Check sheet for the modelled part. Datum: model origin and axes. Units: mm. Face numbers are marked on the shaded views. A direction names the side the tool comes from. Round coordinates to 2 decimals unless told otherwise and drop trailing zeros. Write each loop counter-clockwise with the first axis right and the second up, starting at its lowest first coordinate (ties: lowest second). Pieces come first, ordered by that corner, then holes.
Item 1: Cross-section at D-D on z = -4.5. Enter the section's corners in (x, y).
Item 2: Material ranges on line 1 (Y direction, x = 0.5, z = 0); line 2 (X direction, y = -3.5, z = -0.5); line 3 (Y direction, x = 0, z = -1.25), recorded low to high.
Item 3: Tool access check on the marked faces 4, 5 and 6. Record the directions out of +Z, -Z, +X, -X, +Y, -Y that give a thin tool (end or side, any length) a straight path to the whole face; none if there is none.
Item 4: Cross-section at C-C on x = 6.25. Enter the section's corners in (y, z), plus the area to 3 significant figures.
Item 5: Cross-section at A-A on y = -18.4. Enter the section's corners in (x, z), plus the area to 3 significant figures.
Item 6: Release check for a two-part mould opening along Z. For the marked faces 1, 2 and 3 record: +Z half, -Z half, draft (parallel to the pull), parting line (faces both ways), or undercut.
Item 7: Go/stop test with flat-tipped pins: pin 1 Ø1.6 at (x, z) = (-0.5, 0.5) entering from +Y; pin 2 Ø1.6 at (x, y) = (-0.5, -14) entering from +Z; pin 3 Ø1.6 at (x, y) = (0, -21.5) entering from -Z. Record where each tip stops, or that it passes through.
Item 8: Cross-section at B-B on z = 0. Enter the section's corners in (x, y), plus the area to 3 significant figures.
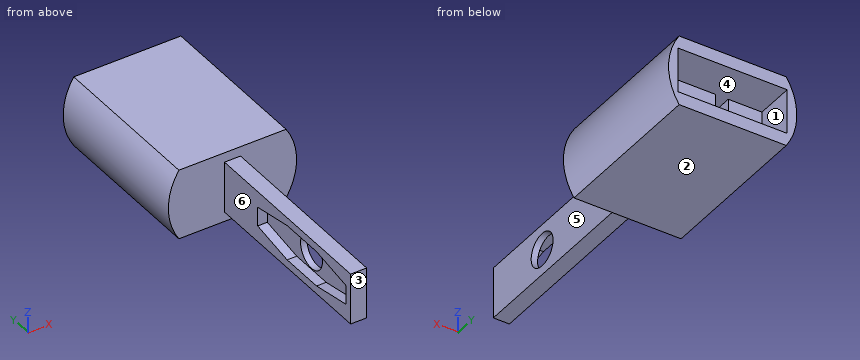
from build123d import *

# Parameters (mm, degrees)
SKETCH3_R           = 10
BOSS_EXTRUDE1_DEPTH = 25
SKETCH4_W           = 2.5
SKETCH4_H           = 8
BOSS_EXTRUDE2_DEPTH = 30
CUT_EXTRUDE1_REACH  = 35.564
SKETCH5_R           = 2.6
SKETCH7_W           = 17
SKETCH7_H           = 7
CUT_EXTRUDE3_DEPTH  = 6
SKETCH8_W           = 2
SKETCH8_H           = 7
CUT_EXTRUDE4_DEPTH  = 4
SKETCH11_W          = 5.5
SKETCH11_H          = 21
CUT_EXTRUDE7_DEPTH  = 1.5
CUT_EXTRUDE5_DEPTH  = 43
BOSS_EXTRUDE3_DEPTH = 1.5


with BuildPart() as part:
    # Sketch3 → Boss-Extrude1 (new body)
    with BuildSketch(Plane(origin=(0, 0, 0), x_dir=(1, 0, 0), z_dir=(0, 1, 0))):
        with Locations(Location((0, 0, 0), (0, 0, 270))):
            Circle(SKETCH3_R)
    extrude(amount=BOSS_EXTRUDE1_DEPTH)

    # Sketch4 → Boss-Extrude2 (add)
    with BuildSketch(Plane(origin=(0, 0, 0), x_dir=(-1, 0, 0), z_dir=(0, -1, 0))):
        Rectangle(SKETCH4_W, SKETCH4_H)
    extrude(amount=BOSS_EXTRUDE2_DEPTH)

    # Sketch5 → Cut-Extrude1 (cut, up to next)
    with BuildSketch(Plane(origin=(1.25, 0, 0), x_dir=(0, 0, -1), z_dir=(1, 0, 0)), mode=Mode.PRIVATE) as cut_extrude1_sk1:
        with Locations((0, -18.4)):
            Circle(SKETCH5_R)
    cut_extrude1_tool1 = extrude(cut_extrude1_sk1.sketch, amount=-CUT_EXTRUDE1_REACH, mode=Mode.PRIVATE) & part.part
    add(cut_extrude1_tool1.solids().sort_by_distance((1.25, -18.4, 0))[0], mode=Mode.SUBTRACT)

    # Sketch7 → Cut-Extrude3 (cut)
    with BuildSketch(Plane(origin=(0, 25, 0), x_dir=(1, 0, 0), z_dir=(0, 1, 0))):
        Rectangle(SKETCH7_W, SKETCH7_H)
    extrude(amount=-CUT_EXTRUDE3_DEPTH, mode=Mode.SUBTRACT)

    # Sketch8 → Cut-Extrude4 (cut)
    with BuildSketch(Plane(origin=(0, 19, 0), x_dir=(1, 0, 0), z_dir=(0, 1, 0))):
        with Locations((-2.25, 0)):
            Rectangle(SKETCH8_W, SKETCH8_H)
    extrude(amount=-CUT_EXTRUDE4_DEPTH, mode=Mode.SUBTRACT)

    # Sketch11 → Cut-Extrude7 (cut)
    with BuildSketch(Plane.ZY.offset(1.25)):
        with Locations((0, -18.4)):
            Rectangle(SKETCH11_W, SKETCH11_H)
    extrude(amount=-CUT_EXTRUDE7_DEPTH, mode=Mode.SUBTRACT)

    # Sketch9 → Cut-Extrude5 (cut)
    with BuildSketch(Plane.XZ):
        with BuildLine():
            Line((8.351646544, -5.5), (-8.351646544, -5.5))
            ThreePointArc((-8.351646544, -5.5), (0, -10), (8.351646544, -5.5))
        make_face()
        with BuildLine():
            Line((8.351646544, 5.5), (-8.351646544, 5.5))
            ThreePointArc((-8.351646544, 5.5), (0, 10), (8.351646544, 5.5))
        make_face()
    extrude(amount=-CUT_EXTRUDE5_DEPTH, mode=Mode.SUBTRACT)

    # Sketch10 → Boss-Extrude3 (add)
    with BuildSketch(Plane.ZY.offset(1.25)):
        Polygon((-2.749970665, -28.900023923), (-2.749970665, -21.900023923), (-1.499970665, -28.900023923), align=None)
        Polygon((1.499970665, -28.900023923), (2.749970665, -28.900023923), (2.749970665, -21.900023923), align=None)
        Polygon((2.749970665, -7.899976077), (2.749970665, -14.899976077), (1.499970665, -7.899976077), align=None)
        Polygon((-1.499970665, -7.899976077), (-2.749970665, -7.899976077), (-2.749970665, -14.899976077), align=None)
    extrude(amount=-BOSS_EXTRUDE3_DEPTH)


solid = part.part
Response values:
1. outline: (-8.93, 0) - (8.93, 0) - (8.93, 25) - (-8.93, 25) - close
2. line 1: y = -30 to -21, -15.8 to 19
2. line 2: x = -1.25 to 1.25
2. line 3: y = -30 to -28.9, -7.9 to 19
3. face 4: +Y
3. face 5: +Z, -Z, +X, -Y
3. face 6: +Z, -Z, -X, -Y
4. outline: (0, -5.5) - (25, -5.5) - (25, -3.5) - (19, -3.5) - (19, 3.5) - (25, 3.5) - (25, 5.5) - (0, 5.5) - close
4. area: 233 mm2
5. outline: (-1.25, -4) - (1.25, -4) - (1.25, -2.6) - (0.25, -2.6) - (0.25, -2.75) - (-1.25, -2.75) - close; (-1.25, 2.75) - (0.25, 2.75) - (0.25, 2.6) - (1.25, 2.6) - (1.25, 4) - (-1.25, 4) - close
5. area: 6.55 mm2
6. face 1: undercut
6. face 2: -Z half
6. face 3: draft
7. pin 1: stops at y = 19
7. pin 2: stops at z = 4
7. pin 3: stops at z = -4
8. outline: (-10, 0) - (-1.25, 0) - (-1.25, -7.9) - (0.25, -7.9) - (0.25, -15.8) - (1.25, -15.8) - (1.25, 0) - (10, 0) - (10, 25) - (8.5, 25) - (8.5, 19) - (-1.25, 19) - (-1.25, 15) - (-3.25, 15) - (-3.25, 19) - (-8.5, 19) - (-8.5, 25) - (-10, 25) - close; (-1.25, -30) - (1.25, -30) - (1.25, -21) - (0.25, -21) - (0.25, -28.9) - (-1.25, -28.9) - close
8. area: 428 mm2
